The listing builds one solid part. Answer for the finished solid, in the listing's coordinates (mm). Round coordinates to 2 decimals unless told otherwise and drop trailing zeros. Order: outer loops, then holes, each group sorted by start corner. A loop starts at its lowest first (then second) coordinate and runs counter-clockwise, first axis right, second up. Notation, with made-up numbers: (36.25, -1) -> (75.25, -1) arc R13 cw to (75.25, 3) -> close; hole circle Ø11 at (76.25, 15). An arc over 180 degrees is marked (long way). Answer in a Markdown table with one row per item. Add a question column.
```python
from build123d import *

# Parameters (mm, degrees)
F1_DEPTH = 6.35
F2_R     = 5.08


with BuildPart() as f1:
    # F0 (on Right) → F1 (new body)
    with BuildSketch(Plane.YZ):
        with BuildLine():
            Line((-44.537589, -10.444656), (-44.537589, 10.247586))
            ThreePointArc((-44.537589, 10.247586), (-54.88371, -0.098535), (-44.537589, -10.444656))
        make_face()
        with BuildLine():
            ThreePointArc((-34.191468, -0.098535), (-37.221777, 7.217278), (-44.537589, 10.247586))
            Line((-44.537589, 10.247586), (-44.537589, -10.444656))
            ThreePointArc((-44.537589, -10.444656), (-37.221777, -7.414347), (-34.191468, -0.098535))
        make_face()
        with BuildLine():
            ThreePointArc((54.489574, -0.098535), (51.459266, 7.217278), (44.143453, 10.247586))
            Line((44.143453, 10.247586), (44.143453, -10.444656))
            ThreePointArc((44.143453, -10.444656), (51.459266, -7.414347), (54.489574, -0.098535))
        make_face()
        with BuildLine():
            Line((44.143453, -10.444656), (44.143453, 10.247586))
            ThreePointArc((44.143453, 10.247586), (33.797332, -0.098535), (44.143453, -10.444656))
        make_face()
        with BuildLine():
            Line((44.143453, 10.247586), (-44.537589, 10.247586))
            ThreePointArc((-44.537589, 10.247586), (-37.221777, 7.217278), (-34.191468, -0.098535))
            ThreePointArc((-34.191468, -0.098535), (-37.221777, -7.414347), (-44.537589, -10.444656))
            Line((-44.537589, -10.444656), (44.143453, -10.444656))
            ThreePointArc((44.143453, -10.444656), (33.797332, -0.098535), (44.143453, 10.247586))
        make_face()
    extrude(amount=F1_DEPTH)

    # F2
    f2_edges = [f1.edges().sort_by_distance(p)[0] for p in [
        (6.35, 54.489574, -0.098535),
        (6.35, -0.197068, 10.247586),
        (6.35, -54.88371, -0.098535),
        (6.35, -0.197068, -10.444656),
    ]]
    fillet(f2_edges, radius=F2_R)


solid = f1.part
```
Item 1: The part is cut by section B-B, the plane x = 3. Give the vertices of the cut face in (y, z), and give its area (3 significant figures).
Item 2: Find the intervals of material crossed by probe 1 along X at (y, z) = (50, -6); probe 2 along Z at (x, y) = (3.5, -10.5); probe 3 along Z at (x, y) = (4.75, 48), in increasing order. Write a range as [from, to].
Item 3: The part is cut by section A-A, the plane y = 20.5. Give the vertices of the cut face in (x, z), and give its area (3 significant figures).
Item 4: For a pull along Y with two mould halves and no side action, classify faces 1 (the face through (0.63, -54.88, 0.13)), 2 (the face through (0, -1, 0)) as released by +Y, released by -Y, zero draft, split by the parting line, or undercut.
Item 5: Flat-ended cylindrical pins translate along their axes: P1, Ø3, axis at y = 37.5, z = -6, coming from the -X side; P2, Ø1, axis at x = 1.5, z = 5.5, coming from the -Y side; P3, Ø2, axis at x = 4, z = -5.5, coming from the +Y side; P4, Ø3, axis at x = 5, y = 12.5, coming from the +Z side. Find the tip coordinate at first contact, or state that the pin passes through.
Resolved:
| question | item | result |
|---|---|---|
| 1 | outline | (-44.54, -10.14) -> (44.14, -10.14) arc R10.04 ccw to (54.19, -0.1) arc R10.04 ccw to (44.14, 9.94) -> (-44.54, 9.94) arc R10.04 ccw to start |
| 1 | area | 2,100 mm2 |
| 2 | probe 1 | [0, 5.33] |
| 2 | probe 2 | [-9.93, 9.73] |
| 2 | probe 3 | [-8.19, 8] |
| 3 | outline | (0, -10.44) -> (1.27, -10.44) arc R5.08 ccw to (6.35, -5.36) -> (6.35, 5.17) arc R5.08 ccw to (1.27, 10.25) -> (0, 10.25) -> close |
| 3 | area | 120 mm2 |
| 4 | face 1 | released by -Y |
| 4 | face 2 | zero draft |
| 5 | P1 | x = 0 |
| 5 | P2 | y = -53.54 |
| 5 | P3 | y = 52.89 |
| 5 | P4 | z = 9.73 |
